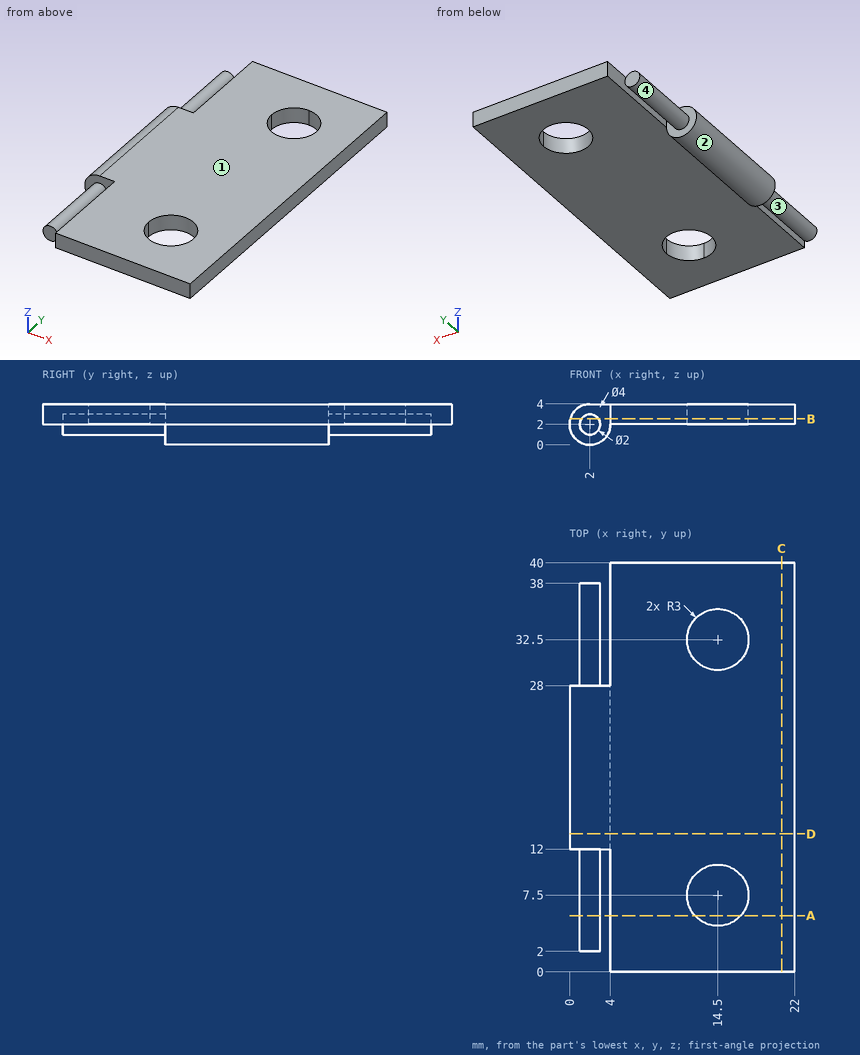
The drawing under review shows one solid part. Ordinate dimensions are in mm from its lowest x, y, z. Round coordinates to 2 decimals unless told otherwise and drop trailing zeros. Write each loop counter-clockwise with the first axis right and the second up, starting at its lowest first coordinate (ties: lowest second). Pieces come first, ordered by that corner, then holes. Notation, with made-up numbers: (51.5, 87) - (109.5, 87) arc R10 ccw to (109.5, 97) - close; hole circle Ø9 at (-21.75, 32.25). An arc over 180 degrees is marked (long way). Use a Markdown table: item, result. Add a question column.
1. We need section D-D (y = 13.5). State the section outline as (x, z) points, then the cut area to 3 significant figures.
2. Clearance check with flat-ended pins moving along their axes: pin 1 (6 mm diameter, centred on x = 18, y = 15, fed in from -Z); pin 2 (1 mm diameter, centred on x = 2.5, z = 2, fed in from +Y); pin 3 (1.2 mm diameter, centred on x = 2, z = 1.5, fed in from -Y); pin 4 (2 mm diameter, centred on x = 13, z = 0.5, fed in from +Y). State where each tip first meets the part, or that it passes through.
3. Wall thickness on probe 1 along X at (y, z) = (5, 2.3); probe 2 along Z at (x, y) = (14.25, 22.5); probe 3 along Z at (x, y) = (2, 37): over which ranges is each line inside the solid? List them lowest first.
4. We need section B-B (z = 2.55). State the section outline as (x, y) points, then the cut area to 3 significant figures.
5. We need section A-A (y = 5.5). State the section outline as (x, z) points, then the cut area to 3 significant figures.
6. We need section C-C (x = 20.75). State the section outline as (y, z) points.
7. Mouldability with a two-part tool opening along X and no side actions: class the marked faces 1, 2, 3 and 4 as +X half, -X half, draft (parallel to the pull), parting line (faces both ways), or undercut.
Output:
| question | item | result |
|---|---|---|
| 1 | outline | (2, 4) arc R2 ccw (long way) to (4, 2) - (22, 2) - (22, 4) - close |
| 1 | area | 49.4 mm2 |
| 2 | pin 1 | stops at z = 2 |
| 2 | pin 2 | stops at y = 38 |
| 2 | pin 3 | stops at y = 2 |
| 2 | pin 4 | passes through |
| 3 | probe 1 | x = 1.05 to 2.95, 4 to 12.84, 16.16 to 22 |
| 3 | probe 2 | z = 2 to 4 |
| 3 | probe 3 | z = 1 to 3 |
| 4 | outline | (0.08, 12) - (1.16, 12) - (1.16, 2) - (2.84, 2) - (2.84, 12) - (4, 12) - (4, 0) - (22, 0) - (22, 40) - (4, 40) - (4, 28) - (2.84, 28) - (2.84, 38) - (1.16, 38) - (1.16, 28) - (0.08, 28) - close; hole circle Ø6 at (14.5, 7.5); hole circle Ø6 at (14.5, 32.5) |
| 4 | area | 760 mm2 |
| 5 | outline | circle Ø2 at (2, 2); (4, 2) - (12.26, 2) - (12.26, 4) - (4, 4) - close; (16.74, 2) - (22, 2) - (22, 4) - (16.74, 4) - close |
| 5 | area | 30.2 mm2 |
| 6 | outline | (0, 2) - (40, 2) - (40, 4) - (0, 4) - close |
| 7 | face 1 | draft |
| 7 | face 2 | parting line |
| 7 | face 3 | undercut |
| 7 | face 4 | undercut |
